Study the drawing (mm; zero at the part's minimum x, y, z) and answer. A direction names the side the tool comes from. Round coordinates to 2 decimals unless told otherwise and drop trailing zeros. Write each loop counter-clockwise with the first axis right and the second up, starting at its lowest first coordinate (ties: lowest second). Pieces come first, ordered by that corner, then holes. Notation, with made-up numbers: (56.25, 0.25) -> (61.25, 0.25) arc R20 ccw to (61.25, 31.25) -> close; hole circle Ø11 at (16.25, -23.75). An arc over 180 degrees is marked (long way). Return JSON: item names as keys, results as strings.
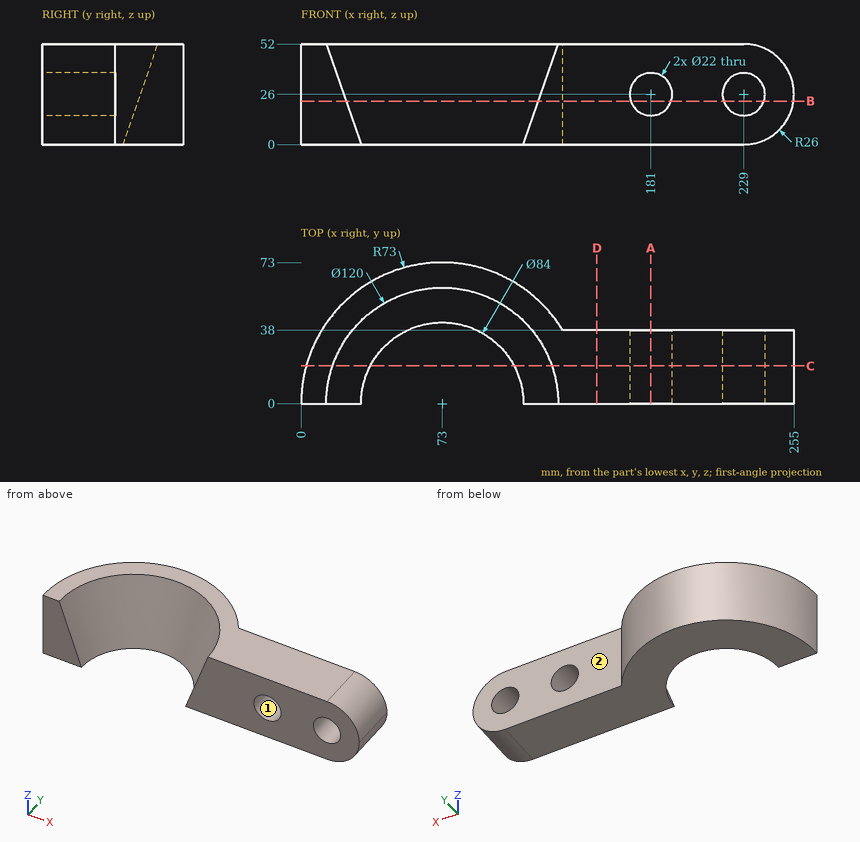
Item 1: A tool of negligible diameter and unlimited length cuts with its end or side. For the marked faces 1 and 2, from which of +Z, -Z, +X, -X, +Y, -Y can it reach the whole face along a straight path? Write none if from no direction.
Worked answers:
{"face 1": "+Y, -Y", "face 2": "+Z, -Z, +X, +Y"}
Item 2: Section C-C (y = 19.5) is taken. State how many separate pieces and enclosed holes the cut face has, then the cut area to 3 significant figures.
Worked answers:
{"separate pieces": "2", "enclosed holes": "2", "area": "7,180 mm2"}
Item 3: Section D-D (x = 153) is taken. Give the vertices of the cut face in (y, z), then the cut area to 3 significant figures.
Worked answers:
{"outline": "(0, 0) -> (38, 0) -> (38, 52) -> (0, 52) -> close", "area": "1,980 mm2"}
Item 4: Section B-B (z = 22.5) is taken. Give the vertices of the cut face in (x, y), then the cut area to 3 significant figures.
Worked answers:
{"outline": "(0, 0) -> (23.21, 0) arc R49.79 cw to (122.79, 0) -> (170.57, 0) -> (170.57, 38) -> (135.33, 38) arc R73 ccw to start; (191.43, 0) -> (218.57, 0) -> (218.57, 38) -> (191.43, 38) -> close; (239.43, 0) -> (254.76, 0) -> (254.76, 38) -> (239.43, 38) -> close", "area": "7,160 mm2"}
Item 5: Straight lines are drawn through the part: L1, parallel to Z at x = 181, y = 28.5; L2, parallel to X at y = 20.5, z = 27; L3, parallel to X at y = 17.5, z = 30.5. For each, find the intervals that lie inside material, in ascending order. Write a range as [from, to].
Worked answers:
{"L1": "z = [0, 15], [37, 52]", "L2": "x = [2.94, 25.92], [120.08, 170.05], [191.95, 218.05], [239.95, 254.98]", "L3": "x = [2.13, 23.44], [122.56, 170.96], [191.04, 218.96], [239.04, 254.61]"}
Item 6: Flat-ended cylindrical pins translate along their axes: pin 1 (6 mm diameter, centred on x = 126, z = 45.5, fed in from +Y); pin 2 (8 mm diameter, centred on y = 53, z = 45, fed in from +X); pin 3 (4 mm diameter, centred on y = 12, z = 8, fed in from +X). Find the tip coordinate at first contact, or state that the pin passes through.
Worked answers:
{"pin 1": "stops at y = 53.19", "pin 2": "stops at x = 127.11", "pin 3": "stops at x = 249.49"}
Item 7: Section A-A (x = 181) is taken. Give the vertices of the cut face in (y, z).
Worked answers:
{"outline": "(0, 0) -> (38, 0) -> (38, 15) -> (0, 15) -> close; (0, 37) -> (38, 37) -> (38, 52) -> (0, 52) -> close"}
